Design review of the part built by this model. Coordinates are the model's own, in mm. Round coordinates to 2 decimals unless told otherwise and drop trailing zeros. Loops run counter-clockwise (first coordinate to the right, second up) from the corner with the lowest first, then second, coordinate; pieces in that order, holes last. Notation, with made-up numbers: M 15,-14.75 L 68,-14.75 A22 cw 68,7.25 Z; hole C 2.5,56.5 d1. An arc over 180 degrees is marked long. One line per item, written item: value. Start each with the question number.
Item 1: We need section A-A (y = 8.5). Write out the cut boundary in (x, z).
Item 2: For line 1 along X through (y, z) = (1.25, -3); line 2 along Z through (x, y) = (152, 9.75); line 3 along X through (y, z) = (3.75, -17.5), list the stretches that pass through material, from the lowest coordinate up.
Item 3: We need section B-B (z = -3). Write out the cut boundary in (x, y), then the cut area to 3 significant figures.
from build123d import *

# Parameters (mm, degrees)
CROQUIS1_W              = 720
CROQUIS1_H              = 200
SALIENTE_EXTRUIR1_DEPTH = 10
CROQUIS2_W              = 20
CROQUIS2_H              = 40
CORTAR_EXTRUIR1_DEPTH   = 10
CROQUIS3_W              = 60
CROQUIS3_H              = 30
CORTAR_EXTRUIR2_DEPTH   = 10


with BuildPart() as part:
    # Croquis1 → Saliente-Extruir1 (new body)
    with BuildSketch(Plane(origin=(0, 0, 0), x_dir=(1, 0, 0), z_dir=(0, 1, 0))):
        Rectangle(CROQUIS1_W, CROQUIS1_H)
    extrude(amount=SALIENTE_EXTRUIR1_DEPTH)

    # Croquis2 → Cortar-Extruir1 (cut)
    with BuildSketch(Plane(origin=(0, 0, 0), x_dir=(-1, 0, 0), z_dir=(0, -1, 0))):
        with Locations((-240, 0)):
            Rectangle(CROQUIS2_W, CROQUIS2_H)
    extrude(amount=-CORTAR_EXTRUIR1_DEPTH, mode=Mode.SUBTRACT)

    # Croquis3 → Cortar-Extruir2 (cut)
    with BuildSketch(Plane(origin=(0, 10, 0), x_dir=(1, 0, 0), z_dir=(0, 1, 0))):
        with Locations((170.145843921, 1.815492006)):
            Rectangle(CROQUIS3_W, CROQUIS3_H)
    extrude(amount=-CORTAR_EXTRUIR2_DEPTH, mode=Mode.SUBTRACT)


solid = part.part
A:
1. outline: M -360,-100 L 360,-100 L 360,100 L -360,100 Z; hole M 140.15,-16.82 L 200.15,-16.82 L 200.15,13.18 L 140.15,13.18 Z; hole M 230,-20 L 250,-20 L 250,20 L 230,20 Z
2. line 1: -360 to 140.15, 200.15 to 230, 250 to 360
2. line 2: -100 to -16.82, 13.18 to 100
2. line 3: -360 to 230, 250 to 360
3. outline: M -360,0 L 140.15,0 L 140.15,10 L -360,10 Z; M 200.15,0 L 230,0 L 230,10 L 200.15,10 Z; M 250,0 L 360,0 L 360,10 L 250,10 Z
3. area: 6,400 mm2
